Autodesk Inventor part; units mm, degrees
ref_plane "to_rring_1_XY" through (2.425, 0, 0) normal (1, 0, 0) x (0, 0, -1)
ref_plane "to_rring_1_YZ" through (2.425, 0, 0) normal (0, 0, -1) x (0, 1, 0)
ref_plane "to_rring_1_ZX" through (2.425, 0, 0) normal (0, 1, 0) x (1, 0, 0)
sketch "Sketch_1" plane through (0, 0, 0) normal (0, 1, 0) x (-1, 0, 0)
  line L0 (-144, 0) -> (0, 0)
  line L1 (0, 0) -> (0, -4.5)
  line L2 (0, -4.5) -> (-0.5, -5)
  line L3 (-0.5, -5) -> (-143.5, -5)
  line L4 (-143.5, -5) -> (-144, -4.5)
  line L5 (-144, -4.5) -> (-144, 0)
  line L6 (-144, 0) -> (0, 0)
revolve "Revolution1" add sketch "Sketch_1" angle 360 about axis through (144, 0, 0) along (1, 0, 0)
sketch "Sketch_27" plane through (0, 0, 0) normal (0, 0, 1) x (1, 0, 0)
  line L0 (144, 0) -> (-144, 0)
  line L1 (1.85, 9.6) -> (1.85, 4.8)
  line L2 (1.85, 4.8) -> (3, 4.8)
  line L3 (3, 4.8) -> (3, 9.6)
  line L4 (3, 9.6) -> (1.85, 9.6)
revolve "Revolution2" cut sketch "Sketch_27" angle 360 about axis through (144, 0, 0) along (1, 0, 0)
sketch "Sketch_39" plane through (0, 0, 0) normal (0, 0, 1) x (1, 0, 0)
  line L0 (144, 0) -> (-144, 0)
  line L1 (138, 9.6) -> (138, 4.8)
  line L2 (138, 4.8) -> (139.15, 4.8)
  line L3 (139.15, 4.8) -> (139.15, 9.6)
  line L4 (139.15, 9.6) -> (138, 9.6)
revolve "Revolution3" cut sketch "Sketch_39" angle 360 about axis through (144, 0, 0) along (1, 0, 0)
sketch "_____7" plane through (0, 0, 5) normal (0, 0, 1) x (1, 0, 0)
  arc A0 (6.5, 1.5) -> (6.5, -1.5) centre (6.5, 0) ccw
  line L0 (6.5, -1.5) -> (21.5, -1.5)
  arc A1 (21.5, -1.5) -> (21.5, 1.5) centre (21.5, 0) ccw
  line L1 (21.5, 1.5) -> (6.5, 1.5)
extrude "Extrusion1" cut sketch "_____7" against normal blind 1.8
sketch "_____10" plane through (0, 0, 5) normal (0, 0, 1) x (1, 0, 0)
  arc A0 (110, 1.5) -> (110, -1.5) centre (110, 0) ccw
  line L0 (110, -1.5) -> (118, -1.5)
  arc A1 (118, -1.5) -> (118, 1.5) centre (118, 0) ccw
  line L1 (118, 1.5) -> (110, 1.5)
extrude "Extrusion2" cut sketch "_____10" against normal blind 1.8
ref_plane "to_rring_1_XY" through (2.425, 0, 0) normal (1, 0, 0) x (0, 0, -1)
ref_plane "to_rring_1_YZ" through (2.425, 0, 0) normal (0, 0, -1) x (0, 1, 0)
ref_plane "to_rring_1_ZX" through (2.425, 0, 0) normal (0, 1, 0) x (1, 0, 0)
ref_plane "to_rring_2_XY" through (138.575, 0, 0) normal (1, 0, 0) x (0, 0, -1)
ref_plane "to_rring_2_YZ" through (138.575, 0, 0) normal (0, 0, -1) x (0, 1, 0)
ref_plane "to_rring_2_ZX" through (138.575, 0, 0) normal (0, 1, 0) x (1, 0, 0)
properties part number "NSFMKRRA10-144-F3-S6-KA5-A18-KB108.5-B11_s"
Geometry check sheet. Reference: the model listing, model coordinates, mm. A direction names the side the tool comes from. Give positions to 0.01 mm unless a question says otherwise; leave off trailing zeros. Order: outer loops, then holes, each group sorted by start corner. A loop starts at its lowest first (then second) coordinate and runs counter-clockwise, first axis right, second up.
1. Gauge pin test, flat ends, axial feed: pin 1 Ø0.5 at (x, z) = (114, 4) entering from -Y; pin 2 Ø0.5 at (x, z) = (15.5, 4) entering from +Y; pin 3 Ø5 at (x, z) = (35, -4) entering from -Y; pin 4 Ø3 at (y, z) = (-0.5, 1) entering from -X. Record the tip position at first contact, or that the pin passes through.
2. Release check for a two-part mould opening along Y. For faces 1 (the face through (144, 0, 0)), 2 (the face through (141.36, -4.88, 1.08)), 3 (the face through (114, 0, 3.2)) record: pulls with the +Y half, pulls with the -Y half, needs draft (parallel to the pull), parting line crosses it, or undercut.
3. Section check C-C, the plane x = 17.5. Enter the section's corners in (y, z), and give its area (3 significant figures).
4. Access from +Z, -Z, +X, -X, +Y, -Y to the whole of each face (thin tool, end or side, straight path). Record for faces 4 (the face through (14, 0, 3.2)), 5 (the face through (71.45, 1.5, -4.77)), 6 (the face through (138.58, 2.58, 4.05)).
5. Section check B-B, the plane x = 54.5. Enter the section's corners in (y, z).
6. Thickness scan on L1, parallel to X at y = -0.5, z = 3.5; L2, parallel to X at y = -4, z = -2.75; L3, parallel to Z at x = 68, y = -3.25. Record the ranges inside material, lowest first.
Values follow:
1. pin 1: stops at y = -3.31
1. pin 2: stops at y = 3.31
1. pin 3: stops at y = -4.77
1. pin 4: stops at x = 0
2. face 1: needs draft
2. face 2: parting line crosses it
2. face 3: undercut
3. outline: (-1.5, 3.2) - (-1.5, 4.77) arc R5 ccw (long way) to (1.5, 4.77) - (1.5, 3.2) - close
3. area: 73.4 mm2
4. face 4: +Z
4. face 5: +X, -X
4. face 6: none
5. outline: circle Ø10 at (0, 0)
6. L1: x = 0 to 5.09, 22.91 to 108.59, 119.41 to 144
6. L2: x = 0.35 to 1.85, 3 to 138, 139.15 to 143.65
6. L3: z = -3.8 to 3.8
